Autodesk Inventor part; units mm, degrees
ref_plane "YZ Plane" through (0, 0, 0) normal (1, 0, 0) x (0, 1, 0)
ref_plane "XZ Plane" through (0, 0, 0) normal (0, 1, 0) x (-1, 0, 0)
ref_plane "XY Plane" through (0, 0, 0) normal (0, 0, 1) x (1, 0, 0)
sketch "Sketch1" plane through (0, 0, 0) normal (0, 1, 0) x (-1, 0, 0)
  circle A0 centre (0, 0) radius 8
  dimension "d0" = 16
extrude "Extrusion1" add sketch "Sketch1" along normal blind 500
sketch "Sketch2" plane through (0, 0, 0) normal (0, -1, 0) x (1, 0, 0)
  circle A0 centre (0, 0) radius 8
extrude "Extrusion2" cut sketch "Sketch2" against normal blind 50
sketch "Sketch3" plane through (0, 50, 0) normal (0, -1, 0) x (1, 0, 0)
  circle A0 centre (0, 0) radius 8
extrude "Extrusion3" add sketch "Sketch3" along normal blind 50
sketch "Sketch4" plane through (0, 0, 0) normal (0, -1, 0) x (1, 0, 0)
  circle A0 centre (0, 0) radius 8
  circle A1 centre (0, 0) radius 6
  dimension "d7" = 12
extrude "Extrusion4" cut sketch "Sketch4" against normal blind 14
thread "Thread1"
sketch "Sketch6" plane through (0, 14, 0) normal (0, -1, 0) x (1, 0, 0)
  circle A0 centre (0, 0) radius 8
  circle A1 centre (0, 0) radius 6.05
  dimension "d13" = 12.1
extrude "Extrusion5" cut sketch "Sketch6" against normal blind 25
sketch "Sketch7" plane through (0, 0, 0) normal (0, -1, 0) x (1, 0, 0)
  circle A0 centre (0, 0) radius 6
  circle A1 centre (0, 0) radius 5
  dimension "d16" = 10
extrude "Extrusion6" add sketch "Sketch7" along normal blind 15 contours A1
sketch "Sketch8" plane through (0, 500, 0) normal (0, 1, 0) x (1, 0, 0)
  circle A0 centre (0, 0) radius 8
extrude "Extrusion7" cut sketch "Sketch8" against normal blind 27.101
sketch "Sketch9" plane through (0, 472.899, 0) normal (0, 1, 0) x (1, 0, 0)
  circle A0 centre (0, 0) radius 8
  circle A1 centre (0, 0) radius 5
  dimension "d21" = 10
extrude "Extrusion8" add sketch "Sketch9" along normal blind 12 contours A1
properties part number "1605_500mm"
Verification items for the finished model (mm, model axes). A direction names the side the tool comes from. Round coordinates to 2 decimals unless told otherwise and drop trailing zeros. Loops run counter-clockwise (first coordinate to the right, second up) from the corner with the lowest first, then second, coordinate; pieces in that order, holes last. Notation, with made-up numbers: (-1.5, -36) - (47.5, -36) arc R31 ccw to (47.5, -10) - close; hole circle Ø1 at (-38.75, -32.75). An arc over 180 degrees is marked (long way). Answer in a Markdown table with one row per item. Add a question column.
Q1. Section check A-A on x = 0. Enter the section's corners in (y, z).
Q2. Section check C-C on y = 168. Enter the section's corners in (x, z).
Q3. Section check B-B on z = 0. Enter the section's corners in (x, y).
Q4. Material ranges on line 1 (X direction, y = 73.5, z = 1); line 2 (X direction, y = 386.5, z = 0.25); line 3 (Y direction, x = 7.25, z = 0), recorded low to high.
Q5. Tool access check on faces 1 (the face through (0, 484.899, 0)), 2 (the face through (-1.08, 478.82, -4.88)), 3 (the face through (-2, 39, 6)). Record the directions out of +Z, -Z, +X, -X, +Y, -Y that give a thin tool (end or side, any length) a straight path to the whole face; none if there is none.
Q6. Gauge pin test, flat ends, axial feed: pin 1 (3 mm diameter, centred on y = 311.5, z = -4.5, fed in from -X); pin 2 (8 mm diameter, centred on y = 37.5, z = -6.5, fed in from +X); pin 3 (4 mm diameter, centred on y = 429.5, z = -3, fed in from +X). Record the tip position at first contact, or that the pin passes through.
Found:
| question | item | result |
|---|---|---|
| 1 | outline | (-15, -5) - (0, -5) - (0, -6) - (14, -6) - (14, -6.05) - (39, -6.05) - (39, -8) - (472.9, -8) - (472.9, -5) - (484.9, -5) - (484.9, 5) - (472.9, 5) - (472.9, 8) - (39, 8) - (39, 6.05) - (14, 6.05) - (14, 6) - (0, 6) - (0, 5) - (-15, 5) - close |
| 2 | outline | circle Ø16 at (0, 0) |
| 3 | outline | (-8, 39) - (-6.05, 39) - (-6.05, 14) - (-6, 14) - (-6, 0) - (-5, 0) - (-5, -15) - (5, -15) - (5, 0) - (6, 0) - (6, 14) - (6.05, 14) - (6.05, 39) - (8, 39) - (8, 472.9) - (5, 472.9) - (5, 484.9) - (-5, 484.9) - (-5, 472.9) - (-8, 472.9) - close |
| 4 | line 1 | x = -7.94 to 7.94 |
| 4 | line 2 | x = -8 to 8 |
| 4 | line 3 | y = 39 to 472.9 |
| 5 | face 1 | +Z, -Z, +X, -X, +Y |
| 5 | face 2 | +Y |
| 5 | face 3 | -Y |
| 6 | pin 1 | stops at x = -7.42 |
| 6 | pin 2 | stops at x = 7.5 |
| 6 | pin 3 | stops at x = 7.94 |
